Part model, mm, in its own coordinate system. Face numbers are marked on the shaded views. Round coordinates to 2 decimals unless told otherwise and drop trailing zeros. Write each loop counter-clockwise with the first axis right and the second up, starting at its lowest first coordinate (ties: lowest second). Pieces come first, ordered by that corner, then holes.
```python
from build123d import *

# Parameters (mm, degrees)
F0_W     = 30
F0_H     = 20
F1_DEPTH = 20
F3_D     = 6.6


with BuildPart() as f1:
    # F0 (on Top) → F1 (new body)
    with BuildSketch(Plane.XY):
        Rectangle(F0_W, F0_H)
    extrude(amount=F1_DEPTH)

    # F3 (through all)
    with Locations(Plane.XY.offset(20)):
        with Locations((-7, 2)):
            Hole(F3_D / 2)

    # F4: F1 across face


with BuildPart() as f1_1:
    add(f1.part)
    add(f1.part.mirror(Plane(origin=(15, 0, 10), x_dir=(0, 1, 0), z_dir=(1, 0, 0))))

    # F5: F1 across face


with BuildPart() as f1_2:
    add(f1_1.part)
    add(f1_1.part.mirror(Plane(origin=(15, -10, 10), x_dir=(1, 0, 0), z_dir=(0, -1, 0))))


solid = f1_2.part
```
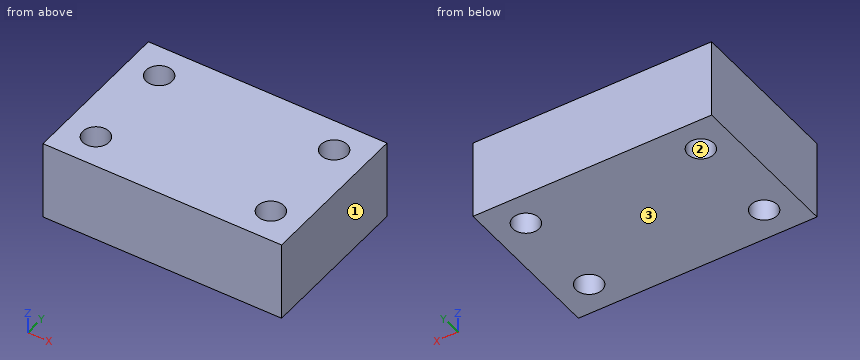
Q1. Mould opens along X. For the marked faces 1, 2 and 3 say: +X half, -X half, draft (parallel to the pull), parting line (faces both ways), or undercut.
Values follow:
face 1: +X half
face 2: undercut
face 3: draft
Q2. Cut at B-B on y = -22. Write the cut outline in (x, z).
Values follow:
outline: (-15, 0) - (-10.3, 0) - (-10.3, 20) - (-15, 20) - close; (-3.7, 0) - (33.7, 0) - (33.7, 20) - (-3.7, 20) - close; (40.3, 0) - (45, 0) - (45, 20) - (40.3, 20) - close
Q3. Cut at A-A on x = 37. Write the cut outline in (y, z).
Values follow:
outline: (-30, 0) - (-25.3, 0) - (-25.3, 20) - (-30, 20) - close; (-18.7, 0) - (-1.3, 0) - (-1.3, 20) - (-18.7, 20) - close; (5.3, 0) - (10, 0) - (10, 20) - (5.3, 20) - close
Q4. Wall check: L1, parallel to X at y = -22, z = 10; L2, parallel to Y at x = 37, z = 12.25; L3, parallel to X at y = -20.5, z = 16.75. Give the ranges that are in metal, low to high.
Values follow:
L1: x = -15 to -10.3, -3.7 to 33.7, 40.3 to 45
L2: y = -30 to -25.3, -18.7 to -1.3, 5.3 to 10
L3: x = -15 to -9.94, -4.06 to 34.06, 39.94 to 45
Q5. Cut at C-C on z = 8. Write the cut outline in (x, y).
Values follow:
outline: (-15, -30) - (45, -30) - (45, 10) - (-15, 10) - close; hole circle Ø6.6 at (-7, -22); hole circle Ø6.6 at (-7, 2); hole circle Ø6.6 at (37, -22); hole circle Ø6.6 at (37, 2)
